For this review, use the dimensioned drawing (mm, ordinates from the lowest corner) and the shaded views. A direction names the side the tool comes from. Give positions to 0.01 mm unless a question says otherwise; leave off trailing zeros. Write each loop counter-clockwise with the first axis right and the second up, starting at its lowest first coordinate (ties: lowest second). Pieces come first, ordered by that corner, then holes. Notation, with made-up numbers: (-4, -30) - (55, -30) arc R23 cw to (55, -11) - close; hole circle Ø10 at (-27.75, 51.5). An arc over 180 degrees is marked (long way). Use a Markdown table: item, result. Add a question column.
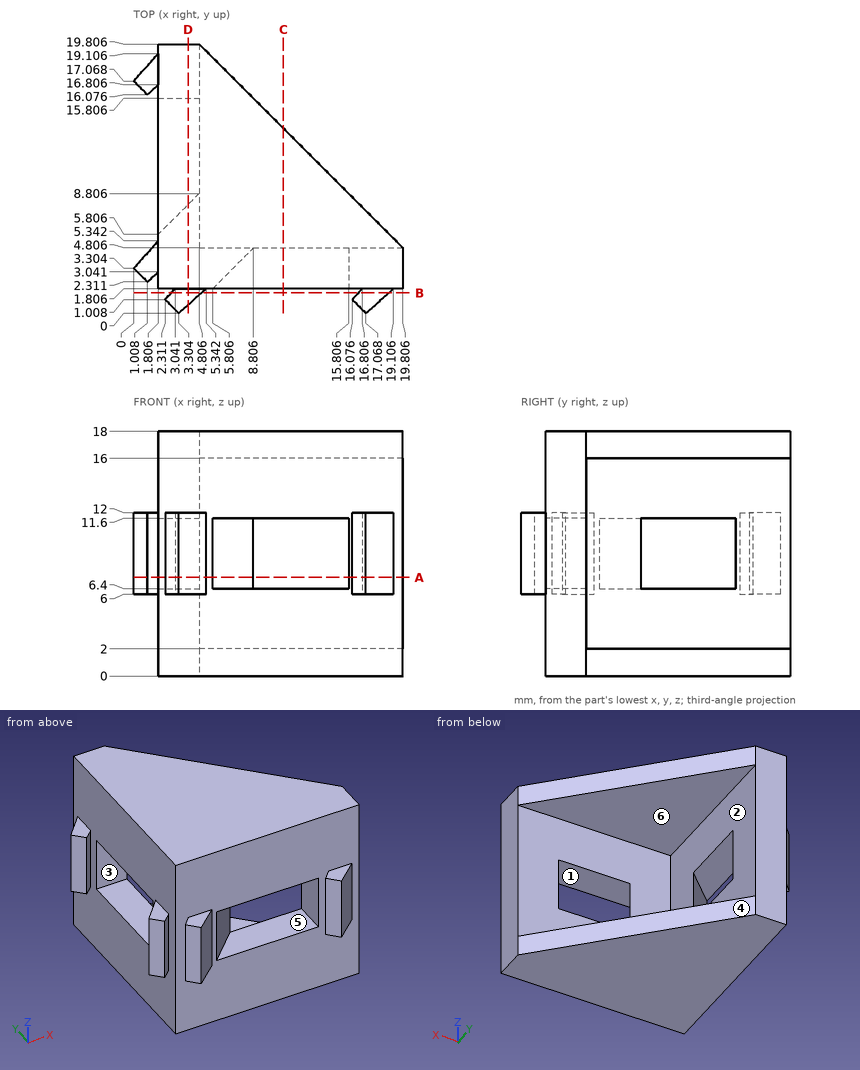
(1) Mouldability with a two-part tool opening along X and no side actions: class the marked faces 4, 5 and 6 as +X half, -X half, draft (parallel to the pull), parting line (faces both ways), or undercut.
(2) Add section B-B (y = 1.5). State the section outline as (x, z) points (1 decimal).
(3) Add section A-A (z = 7.25). Count the separate pieces of the cut face and the enclosed holes in it.
(4) Insertion check: pin 1 (0.5 mm diameter, centred on x = 17, y = 1, fed in from +Z); pin 2 (1.5 mm diameter, centred on x = 7, z = 4, fed in from -Y); pin 3 (3.5 mm diameter, centred on x = 3.5, z = 8.5, fed in from -Y). Each pin has a flat end and moves straight along its axis. Give the tip position at first contact, or say it passes through.
(5) Tool access review of the marked faces 1, 2 and 3: name each direction out of +Z, -Z, +X, -X, +Y, -Y from which nothing blocks a thin tool from reaching the whole face with its end or side.
(6) Add section C-C (x = 11). State the section outline as (y, z) points.
(7) For line 1 along Z through (x, y) = (12.25, 9.75); line 2 along Z through (x, y) = (9.75, 3.5); line 3 along X through (y, z) = (16, 14.5), list the stretches that pass through material, from the lowest coordinate up.
(8) Add section D-D (x = 4). State the section outline as (y, z) points.
Answers follow:
| question | item | result |
|---|---|---|
| 1 | face 4 | +X half |
| 1 | face 5 | undercut |
| 1 | face 6 | draft |
| 2 | outline | (2.8, 6) - (5, 6) - (5, 12) - (2.8, 12) - close; (16.5, 6) - (18.8, 6) - (18.8, 12) - (16.5, 12) - close |
| 3 | separate pieces | 3 |
| 3 | enclosed holes | 0 |
| 4 | pin 1 | z = 12 |
| 4 | pin 2 | y = 1.81 |
| 4 | pin 3 | y = 0 |
| 5 | face 1 | -Y |
| 5 | face 2 | +X, +Y |
| 5 | face 3 | +X, -X |
| 6 | outline | (1.81, 0) - (13.61, 0) - (13.61, 2) - (4.81, 2) - (4.81, 6.4) - (1.81, 6.4) - close; (1.81, 11.6) - (4.81, 11.6) - (4.81, 16) - (13.61, 16) - (13.61, 18) - (1.81, 18) - close |
| 7 | line 1 | 0 to 2, 16 to 18 |
| 7 | line 2 | 0 to 6.4, 11.6 to 18 |
| 7 | line 3 | 1.81 to 4.81 |
| 8 | outline | (0.62, 6) - (1.81, 6) - (1.81, 0) - (19.81, 0) - (19.81, 18) - (1.81, 18) - (1.81, 12) - (0.62, 12) - close; hole (8, 6.4) - (15.81, 6.4) - (15.81, 11.6) - (8, 11.6) - close |
